Here's how the part is built. I have some questions about the finished solid (model axes, mm). A direction names the side the tool comes from. Coordinates: 2 decimals unless noted, no trailing zeros. Write each loop counter-clockwise with the first axis right and the second up, starting at its lowest first coordinate (ties: lowest second). Pieces come first, ordered by that corner, then holes. Notation, with made-up numbers: (-15.5, 14.5) -> (-4.5, 14.5) arc R31 ccw to (-4.5, 38.5) -> close; hole circle Ø11 at (37, 49.5). An arc over 180 degrees is marked (long way). Put each result on its own line as item: value.
```python
from build123d import *

# Parameters (mm, degrees)
SKETCH2_R           = 1.075
SKETCH2_R_2         = 2.75
BOSS_EXTRUDE1_DEPTH = 5.15
SHELL1_T            = -1.1


with BuildPart() as part:
    # Sketch2 → Boss-Extrude1 (new body)
    with BuildSketch(Plane(origin=(0, 0, 0), x_dir=(1, 0, 0), z_dir=(0, 1, 0))):
        with BuildLine():
            Line((0, 11.1), (20, 11.1))
            Line((20, 11.1), (20, -11.1))
            Line((20, -11.1), (0, -11.1))
            ThreePointArc((0, -11.1), (-11.1, 0), (0, 11.1))
        make_face()
        with Locations(Location((-4.242640687, 4.242640687, 0), (0, 0, 90))):
            Circle(SKETCH2_R, mode=Mode.SUBTRACT)
        with Locations(Location((4.242640687, 4.242640687, 0), (0, 0, 90))):
            Circle(SKETCH2_R, mode=Mode.SUBTRACT)
        with Locations(Location((-4.242640687, -4.242640687, 0), (0, 0, 90))):
            Circle(SKETCH2_R, mode=Mode.SUBTRACT)
        with Locations(Location((4.242640687, -4.242640687, 0), (0, 0, 90))):
            Circle(SKETCH2_R, mode=Mode.SUBTRACT)
        with Locations(Location((0, 0, 0), (0, 0, 90))):
            Circle(SKETCH2_R_2, mode=Mode.SUBTRACT)
    extrude(amount=BOSS_EXTRUDE1_DEPTH)

    # Shell1
    shell1_openings = [part.faces().sort_by_distance(p)[0] for p in [
        (20, 2.575, 0),
    ]]
    offset(amount=SHELL1_T, openings=shell1_openings)


solid = part.part
```
Item 1: Imagine slicing it at C-C on y = 2.55. Write out the boundary of the cut face in (x, z) (3 decimals), then the cut area to 3 significant figures.
Output:
outline: (-2.902, -2.53) arc R2.175 ccw (long way) to (-2.53, -2.902) arc R3.85 ccw to (2.53, -2.902) arc R2.175 ccw (long way) to (2.902, -2.53) arc R3.85 ccw to (2.902, 2.53) arc R2.175 ccw (long way) to (2.53, 2.902) arc R3.85 ccw to (-2.53, 2.902) arc R2.175 ccw (long way) to (-2.902, 2.53) arc R3.85 ccw to start; (0, -11.1) -> (20, -11.1) -> (20, -10) -> (0, -10) arc R10 cw to (0, 10) -> (20, 10) -> (20, 11.1) -> (0, 11.1) arc R11.1 ccw to start; hole circle Ø2.15 at (-4.243, -4.243); hole circle Ø2.15 at (-4.243, 4.243); hole circle Ø5.5 at (0, 0); hole circle Ø2.15 at (4.243, -4.243); hole circle Ø2.15 at (4.243, 4.243)
area: 148 mm²
Item 2: If we mould it in two halves opening along Z, with no side actions, what happens to faces 1 (the flat face through (5, 0, 0)), 2 (the cylindrical face through (4.195, 2.539, 5.317)), 3 (the flat face through (10, 3, 11.1))? For each: released by +Z, released by -Z, zero draft, split by the parting line, or undercut.
Output:
face 1: zero draft
face 2: undercut
face 3: released by +Z
Item 3: For P1, Ø1.5, axis at y = 2.5, z = -3, coming from the +X side; P2, Ø1.9, axis at x = 4.24, z = -4.24, coming from the -Y side; P3, Ø1.5, axis at y = 3, z = 4, coming from the -X side, each with a flat end and sliding along its axis, tell me the tip position at first contact or that it passes through.
Output:
P1: stops at x = 6.36
P2: passes through
P3: stops at x = -10.61
Item 4: Imagine slicing it at A-A on z = 0. Write out the boundary of the cut face in (x, y).
Output:
outline: (-11.1, 0) -> (-2.75, 0) -> (-2.75, 5.15) -> (-11.1, 5.15) -> close; (2.75, 0) -> (20, 0) -> (20, 1.1) -> (3.85, 1.1) -> (3.85, 4.05) -> (20, 4.05) -> (20, 5.15) -> (2.75, 5.15) -> close; hole (-10, 1.1) -> (-3.85, 1.1) -> (-3.85, 4.05) -> (-10, 4.05) -> close
Item 5: Imagine slicing it at D-D on x = -9. Write out the boundary of the cut face in (y, z).
Output:
outline: (0, -6.5) -> (5.15, -6.5) -> (5.15, 6.5) -> (0, 6.5) -> close; hole (1.1, -4.36) -> (4.05, -4.36) -> (4.05, 4.36) -> (1.1, 4.36) -> close
Item 6: Which directions (+Z, -Z, +X, -X, +Y, -Y) give clear straight access to the entire face, cutting with the end or side of a thin tool? Please do faces 4 (the flat face through (10, 3, -10)), 5 (the cylindrical face through (-4.969, 2.539, 5.035)), 6 (the cylindrical face through (-10, 3, 0)).
Output:
face 4: +X
face 5: +Y, -Y
face 6: none
Item 7: Please list where these lines run through material, in increasing order: line 1 along Z through (x, y) = (15, 2.85); line 2 along Y through (x, z) = (2, -4); line 3 along X through (y, z) = (2.9, -6). Write a range as from..to.
Output:
line 1: z = -11.1..-10, 10..11.1
line 2: y = 0..1.1, 4.05..5.15
line 3: x = -9.34..-8, -5.52..-2.96, 2.96..5.52
Item 8: Imagine slicing it at B-B on x = 8.5. Write out the boundary of the cut face in (y, z), then the cut area to 3 significant figures.
Output:
outline: (0, -11.1) -> (5.15, -11.1) -> (5.15, 11.1) -> (0, 11.1) -> close; hole (1.1, -10) -> (4.05, -10) -> (4.05, 10) -> (1.1, 10) -> close
area: 55.3 mm²
